For this review, take the finished solid that the model builds, in its own axes (mm). A direction names the side the tool comes from. Coordinates: 2 decimals unless noted, no trailing zeros. Write each loop counter-clockwise with the first axis right and the second up, starting at its lowest first coordinate (ties: lowest second). Pieces come first, ordered by that corner, then holes.
1) Mouldability with a two-part tool opening along X and no side actions: class faces 1 (the face through (65, -16.2, -1.5)), 2 (the face through (3.981, -26.846, -5.961)), 3 (the face through (-25.75, -27, 0)), 4 (the face through (-24.764, 22.345, 14.246)) as pulls with the +X half, pulls with the -X half, needs draft (parallel to the pull), parting line crosses it, or undercut.
2) Insertion check: P1, Ø8, axis at x = -45.5, z = -16, coming from the +Y side; P2, Ø5, axis at x = 4.5, z = 13.5, coming from the +Y side; P3, Ø5, axis at x = -43, z = 4, coming from the -Y side; P4, Ø15, axis at y = 5.5, z = -2.5, coming from the +X side. Each pin has a flat end and moves straight along its axis. Give the tip position at first contact, or say it passes through.
3) We need section C-C on x = -46.5. Write out the cut boundary in (y, z), then the cut area to 3 significant figures.
4) We need section A-A on z = 0. Write out the cut boundary in (x, y), then the cut area to 3 significant figures.
5) For faces 5 (the face through (50, 10, -13)), 6 (the face through (-23.75, 23, -14)), 7 (the face through (59.17, -21.477, -4.769)), list the 3-axis set-ups (+Z, -Z, +X, -X, +Y, -Y) from which the entire face can be reached by the end or side of a thin tool; tool diameter is ignored.
6) To check wall thickness, follow line 1 along X through (y, z) = (5.5, -15.5); line 2 along Y through (x, z) = (-28, 8); line 3 along X through (y, z) = (-20, -20). State the ranges of each line that lie inside material, in increasing order.
from build123d import *

# Parameters (mm, degrees)
F2_R     = 16
F3_DEPTH = 130
F4_R     = 19
F5_DEPTH = 115


with BuildPart() as f1:
    # F0 (on Front) → F1 (revolve)
    with BuildSketch(Plane.XZ):
        Polygon((-65, 30), (-65, 0), (65, 0), (65, 22), (53.5, 22), (53.5, 25), (35.5, 25), (32.5, 27.5), (-23.75, 27.5), (-23.75, 26.5), (-25.75, 26.5), (-25.75, 30), align=None)
    revolve(axis=Axis((0, 0, 0), (-1, 0, 0)))

    # F2 (on face) → F3 (cut, through all)
    with BuildSketch(Plane.YZ.offset(65)):
        Circle(F2_R)
    extrude(amount=-F3_DEPTH, mode=Mode.SUBTRACT)

    # F4 (on face) → F5 (cut)
    with BuildSketch(Plane(origin=(-65, 0, 0), x_dir=(0, -1, 0), z_dir=(-1, 0, 0))):
        Circle(F4_R)
    extrude(amount=-F5_DEPTH, mode=Mode.SUBTRACT)


solid = f1.part
Result:
1. face 1: pulls with the +X half
1. face 2: needs draft
1. face 3: undercut
1. face 4: undercut
2. P1: stops at y = 27.5
2. P2: stops at y = 25.2
2. P3: stops at y = -29.96
2. P4: passes through
3. outline: circle Ø60 at (0, 0); hole circle Ø38 at (0, 0)
3. area: 1,690 mm2
4. outline: (-65, -30) - (-25.75, -30) - (-25.75, -26.5) - (-23.75, -26.5) - (-23.75, -27.5) - (32.5, -27.5) - (35.5, -25) - (53.5, -25) - (53.5, -22) - (65, -22) - (65, -16) - (50, -16) - (50, -19) - (-65, -19) - close; (-65, 19) - (50, 19) - (50, 16) - (65, 16) - (65, 22) - (53.5, 22) - (53.5, 25) - (35.5, 25) - (32.5, 27.5) - (-23.75, 27.5) - (-23.75, 26.5) - (-25.75, 26.5) - (-25.75, 30) - (-65, 30) - close
4. area: 2,270 mm2
5. face 5: -X
5. face 6: none
5. face 7: +X
6. line 1: x = 50 to 65
6. line 2: y = -28.91 to -17.23, 17.23 to 28.91
6. line 3: x = -65 to -25.75
